The listing builds one solid part. Answer for the finished solid, in the listing's coordinates (mm). Round coordinates to 2 decimals unless told otherwise and drop trailing zeros. Write each loop counter-clockwise with the first axis right and the second up, starting at its lowest first coordinate (ties: lowest second). Pieces come first, ordered by that corner, then holes. Notation, with made-up numbers: (33.5, 23) - (72.5, 23) arc R35 ccw to (72.5, 56) - close; hole circle Ø1 at (85, 66.25). An arc over 180 degrees is marked (long way). Use a Markdown table: item, result. Add a question column.
1) A cutting plane is placed at A-A (y = 2.25). Give the vertices of the cut face in (x, z), then the cut area to 3 significant figures.
2) Each of these flat-tipped pins is pushed along its axis until it touches: P1, Ø1, axis at y = 2, z = -76, coming from the -X side; P2, Ø1.6, axis at x = -57.5, y = 1.5, coming from the -Z side; P3, Ø1.6, axis at x = 135, y = 1, coming from the +Z side; P4, Ø6.5, axis at x = 127.96, z = -30.8, coming from the -Y side. Where does it stop, or does it pass through?
3) A cutting plane is placed at B-B (x = -19.5). Give the vertices of the cut face in (y, z) (3 decimals).
4) Find the intervals of material crossed by probe 1 along Z at (x, y) = (129, 1.9); probe 2 along Z at (x, y) = (123.5, 2.7); probe 3 along X at (y, z) = (2.3, -12), in increasing order. Write a range as from..to.
5) Determine the mould class of faces 1 (the cylindrical face through (125.93, 1.57, -30.89)), 2 (the flat face through (41, 3.175, -12)) for opening direction Z: +Z half, -Z half, draft (parallel to the pull), parting line (faces both ways), or undercut.
```python
from build123d import *

# Parameters (mm, degrees)
SKETCH1_W           = 203.2
SKETCH1_H           = 127
SKETCH1_R           = 2.032
BOSS_EXTRUDE1_DEPTH = 3.175
SKETCH5_W           = 25.4
SKETCH5_H           = 3.175
BOSS_EXTRUDE2_DEPTH = 3.175
SKETCH6_W           = 25.4
SKETCH6_H           = 3.175
BOSS_EXTRUDE3_DEPTH = 3.175
SKETCH7_W           = 25.908
SKETCH7_H           = 3.175
CUT_EXTRUDE1_DEPTH  = 3.175


with BuildPart() as part:
    # Sketch1 → Boss-Extrude1 (new body)
    with BuildSketch(Plane(origin=(0, 0, 0), x_dir=(1, 0, 0), z_dir=(0, 1, 0))):
        with Locations((42.361845493, 11.49358269)):
            Rectangle(SKETCH1_W, SKETCH1_H)
        with Locations((127.959845493, -7.93741731)):
            Circle(SKETCH1_R, mode=Mode.SUBTRACT)
        with Locations((127.959845493, 30.79758269)):
            Circle(SKETCH1_R, mode=Mode.SUBTRACT)
    extrude(amount=BOSS_EXTRUDE1_DEPTH)

    # Sketch5 → Boss-Extrude2 (add)
    with BuildSketch(Plane.XY.offset(52.00641731)):
        with Locations((16.961845493, 1.5875)):
            Rectangle(SKETCH5_W, SKETCH5_H)
        with Locations((105.861845493, 1.5875)):
            Rectangle(SKETCH5_W, SKETCH5_H)
    extrude(amount=BOSS_EXTRUDE2_DEPTH)

    # Sketch6 → Boss-Extrude3 (add)
    with BuildSketch(Plane(origin=(0, 0, -74.99358269), x_dir=(-1, 0, 0), z_dir=(0, 0, -1))):
        with Locations((-105.861845493, 1.5875)):
            Rectangle(SKETCH6_W, SKETCH6_H)
        with Locations((-16.961845493, 1.5875)):
            Rectangle(SKETCH6_W, SKETCH6_H)
    extrude(amount=BOSS_EXTRUDE3_DEPTH)

    # Sketch7 → Cut-Extrude1 (cut)
    with BuildSketch(Plane.ZY.offset(59.238154507)):
        with Locations((-11.49358269, 1.5875)):
            Rectangle(SKETCH7_W, SKETCH7_H)
    extrude(amount=-CUT_EXTRUDE1_DEPTH, mode=Mode.SUBTRACT)


solid = part.part
```
Entries:
| question | item | result |
|---|---|---|
| 1 | outline | (-59.24, -74.99) - (4.26, -74.99) - (4.26, -78.17) - (29.66, -78.17) - (29.66, -74.99) - (93.16, -74.99) - (93.16, -78.17) - (118.56, -78.17) - (118.56, -74.99) - (143.96, -74.99) - (143.96, 52.01) - (118.56, 52.01) - (118.56, 55.18) - (93.16, 55.18) - (93.16, 52.01) - (29.66, 52.01) - (29.66, 55.18) - (4.26, 55.18) - (4.26, 52.01) - (-59.24, 52.01) - (-59.24, 1.46) - (-56.06, 1.46) - (-56.06, -24.45) - (-59.24, -24.45) - close; hole circle Ø4.06 at (127.96, -30.8); hole circle Ø4.06 at (127.96, 7.94) |
| 1 | area | 26,000 mm² |
| 2 | P1 | stops at x = 4.26 |
| 2 | P2 | stops at z = -74.99 |
| 2 | P3 | stops at z = 52.01 |
| 2 | P4 | stops at y = 0 |
| 3 | outline | (0, -74.994) - (3.175, -74.994) - (3.175, 52.006) - (0, 52.006) - close |
| 4 | probe 1 | z = -74.99..-32.54, -29.05..6.19, 9.68..52.01 |
| 4 | probe 2 | z = -74.99..52.01 |
| 4 | probe 3 | x = -56.06..143.96 |
| 5 | face 1 | undercut |
| 5 | face 2 | draft |
